Here's how the part is built. I have some questions about the finished solid (model axes, mm). Face numbers are marked on the shaded views. A direction names the side the tool comes from. Round coordinates to 2 decimals unless told otherwise and drop trailing zeros. Order: outer loops, then holes, each group sorted by start corner. A loop starts at its lowest first (then second) coordinate and runs counter-clockwise, first axis right, second up. Notation, with made-up numbers: M -10,75.25 L 34,75.25 A25 ccw 34,96.25 Z; hole C 4.5,25.25 d6. An arc over 180 degrees is marked long. Write item = value, one per line. Start each with the question number.
Item 1: I want a section at B-B, the plane y = 0. List the corners of the cut face in (x, z) for me (3 decimals).
Item 2: I'm going to push flat-ended pins straight in: P1, Ø3, axis at x = 12, z = 29, coming from the -Y side; P2, Ø5, axis at x = 60, y = -43, coming from the +Z side; P3, Ø5, axis at x = 31, z = 25, coming from the +Y side. Where does each tip first touch, or does it pass through?
Item 3: I want a section at C-C, the plane x = -47. List the corners of the cut face in (y, z) for me (3 decimals), plus the area to 3 significant figures.
Item 4: Please list where these lines run through material, in increasing order: L1, parallel to Z at x = -30, y = -37.5; L2, parallel to Y at x = 10.5, z = 88; L3, parallel to X at y = -30, z = 59.
Item 5: I want a section at A-A, the plane x = 0. List the corners of the cut face in (y, z) for me (3 decimals).
Item 6: I want a section at D-D, the plane z = 67.5. List the corners of the cut face in (x, y) for me.
Item 7: For the marked faces 1 and 2, which set-ups out of +Z, -Z, +X, -X, +Y, -Y let a thin tool reach every point of the face, with its end or its side?
```python
from build123d import *

# Parameters (mm, degrees)
F0_W     = 183.617264
F0_H     = 108.108356
F1_DEPTH = 25.4
F2_R     = 6.35
F3_R     = 37.05912
F4_DEPTH = 78.90592
F5_R     = 5.08
F6_R     = 3.175


with BuildPart() as f1:
    # F0 (on Top) → F1 (new body)
    with BuildSketch(Plane.XY):
        Rectangle(F0_W, F0_H)
    extrude(amount=F1_DEPTH)

    # F2
    f2_edges = [f1.edges().sort_by_distance(p)[0] for p in [
        (-91.808632, -54.054178, 12.7),
        (91.808632, -54.054178, 12.7),
        (91.808632, 54.054178, 12.7),
        (-91.808632, 54.054178, 12.7),
    ]]
    fillet(f2_edges, radius=F2_R)

    # F3 (on face) → F4 (join)
    with BuildSketch(Plane.XY.offset(25.4)):
        Circle(F3_R)
    extrude(amount=F4_DEPTH)

    # F5
    f5_edges = [f1.edges().sort_by_distance(p)[0] for p in [
        (37.05912, 0, 64.85296),
        (-37.05912, 0, 25.4),
        (-37.05912, 0, 104.30592),
    ]]
    fillet(f5_edges, radius=F5_R)

    # F6
    f6_edges = [f1.edges().sort_by_distance(p)[0] for p in [
        (-31.97912, 0, 104.30592),
        (-91.808632, 0, 25.4),
    ]]
    fillet(f6_edges, radius=F6_R)


solid = f1.part
```
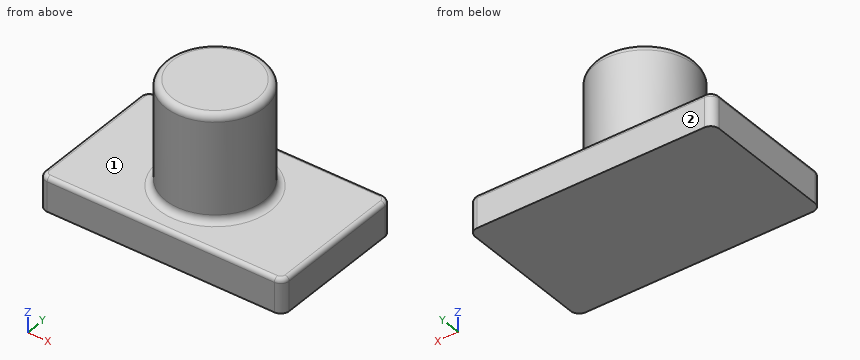
Filled in:
q1.outline = M -91.809,0 L 91.809,0 L 91.809,22.225 A3.175 ccw 88.634,25.4 L 42.139,25.4 A5.08 cw 37.059,30.48 L 37.059,99.226 A5.08 ccw 31.979,104.306 L -31.979,104.306 A5.08 ccw -37.059,99.226 L -37.059,30.48 A5.08 cw -42.139,25.4 L -88.634,25.4 A3.175 ccw -91.809,22.225 Z
q2.P1 = -36.18
q2.P2 = 25.4
q2.P3 = 54.04
q3.outline = M -54.054,0 L 54.054,0 L 54.054,22.225 A3.175 ccw 50.879,25.4 L -50.879,25.4 A3.175 ccw -54.054,22.225 Z
q3.area = 2,740 mm^2
q4.L1 = 0 to 25.4
q4.L2 = -35.54 to 35.54
q4.L3 = -21.76 to 21.76
q5.outline = M -54.054,0 L 54.054,0 L 54.054,22.225 A3.175 ccw 50.879,25.4 L 42.139,25.4 A5.08 cw 37.059,30.48 L 37.059,99.226 A5.08 ccw 31.979,104.306 L -31.979,104.306 A5.08 ccw -37.059,99.226 L -37.059,30.48 A5.08 cw -42.139,25.4 L -50.879,25.4 A3.175 ccw -54.054,22.225 Z
q6.outline = C 0,0 d74.12
q7.face_1 = +Z
q7.face_2 = +Z, -Z, +X, -X, +Y
